from build123d import *

# Parameters (mm, degrees)
CROQUIS1_W              = 154.2
CROQUIS1_H              = 154.2
SALIENTE_EXTRUIR1_DEPTH = 0.8
CROQUIS2_R              = 60
CORTAR_EXTRUIR1_DEPTH   = 110.038800434
SALIENTE_EXTRUIR2_START = 1
CROQUIS3_R              = 60.995810587
CROQUIS3_R_2            = 60
SALIENTE_EXTRUIR2_DEPTH = 1
SALIENTE_EXTRUIR3_START = 0.5
CROQUIS4_R              = 62.434019261
CROQUIS4_R_2            = 60
SALIENTE_EXTRUIR3_DEPTH = 0.5
CROQUIS5_R              = 2.5
CROQUIS5_R_2            = 60
CORTAR_EXTRUIR2_DEPTH   = 110.046182877


with BuildPart() as part:
    # Croquis1 → Saliente-Extruir1 (new body)
    with BuildSketch(Plane(origin=(0, 0, 0), x_dir=(1, 0, 0), z_dir=(0, 1, 0))):
        Rectangle(CROQUIS1_W, CROQUIS1_H)
    extrude(amount=SALIENTE_EXTRUIR1_DEPTH)

    # Croquis2 → Cortar-Extruir1 (cut, through all)
    with BuildSketch(Plane(origin=(0, 0.8, 0), x_dir=(1, 0, 0), z_dir=(0, 1, 0))):
        with Locations(Location((0, 0, 0), (0, 0, 270))):
            Circle(CROQUIS2_R)
    extrude(amount=-CORTAR_EXTRUIR1_DEPTH, mode=Mode.SUBTRACT)

    # Croquis3 → Saliente-Extruir2 (add)
    with BuildSketch(Plane(origin=(0, 0.8, 0), x_dir=(1, 0, 0), z_dir=(0, 1, 0)).offset(SALIENTE_EXTRUIR2_START)):
        with Locations(Location((0, 0, 0), (0, 0, 90))):
            Circle(CROQUIS3_R)
        with Locations(Location((0, 0, 0), (0, 0, 270))):
            Circle(CROQUIS3_R_2, mode=Mode.SUBTRACT)
    extrude(amount=-SALIENTE_EXTRUIR2_DEPTH)

    # Croquis4 → Saliente-Extruir3 (add)
    with BuildSketch(Plane(origin=(0, 1.8, 0), x_dir=(1, 0, 0), z_dir=(0, 1, 0)).offset(SALIENTE_EXTRUIR3_START)):
        with Locations(Location((0, 0, 0), (0, 0, 270))):
            Circle(CROQUIS4_R)
        with Locations(Location((0, 0, 0), (0, 0, 270))):
            Circle(CROQUIS4_R_2, mode=Mode.SUBTRACT)
    extrude(amount=-SALIENTE_EXTRUIR3_DEPTH)

    # Croquis5 → Cortar-Extruir2 (cut, through all)
    with BuildSketch(Plane(origin=(0, 0.8, 0), x_dir=(1, 0, 0), z_dir=(0, 1, 0))):
        with Locations(Location((-59.39696962, 59.39696962, 0), (0, 0, 270))):
            Circle(CROQUIS5_R)
        with Locations(Location((-59.39696962, -59.39696962, 0), (0, 0, 90))):
            Circle(CROQUIS5_R)
        with Locations(Location((59.39696962, -59.39696962, 0), (0, 0, 270))):
            Circle(CROQUIS5_R)
        with Locations(Location((0, 0, 0), (0, 0, 270))):
            Circle(CROQUIS5_R_2)
        with Locations(Location((59.39696962, 59.39696962, 0), (0, 0, 90))):
            Circle(CROQUIS5_R)
    extrude(amount=-CORTAR_EXTRUIR2_DEPTH, mode=Mode.SUBTRACT)


solid = part.part
Source: CAD feature listing. Evaluate the final solid. Frame: model axes, mm. A direction names the side the tool comes from. Give positions to 0.01 mm unless a question says otherwise; leave off trailing zeros. Write each loop counter-clockwise with the first axis right and the second up, starting at its lowest first coordinate (ties: lowest second). Pieces come first, ordered by that corner, then holes. Notation, with made-up numbers: M 8.5,57 L 31.5,57 A32 ccw 31.5,90 Z; hole C 76,2.25 d3. An arc over 180 degrees is marked long. Return JSON: item names as keys, results as strings. Group by question number.
1) Draft query along Z for faces 3 (the face through (61.876, 0.406, 59.072)), 4 (the face through (37.12, 1.31, 48.4)), 5 (the face through (-60, 1.8, 14)). Return one class per face: released by +Z, released by -Z, zero draft, split by the parting line, or undercut.
2) Set-up query: faces 1 (the face through (-37.99, 2.053, -49.546)), 2 (the face through (33, 0, -52)). Return all of +Z, -Z, +X, -X, +Y, -Y with unobstructed straight access to the full face (end or side cutting, diameter ignored); none if empty.
3) Cut plane B-B, the plane x = 0. Output: boundary loops of the cut face in (y, z).
4) Ray query, L1, parallel to Z at x = 3.5, y = 1.6; L2, parallel to Z at x = 32.5, y = 1.9; L3, parallel to Y at x = -66.5, z = 22. Return the intervals inside material, ascending.
5) Cut plane A-A, the plane z = 0. Output: boundary loops of the cut face in (x, y), then the cut area to 3 significant figures.
6) First-contact query: pin 1 Ø8 at (x, z) = (-59.4, -59.4) entering from +Y. Flat tip, straight axial feed; report the tip coordinate or a pass-through.
Data:
{
 "1": {"face 3": "undercut", "face 4": "split by the parting line", "face 5": "zero draft"},
 "2": {"face 1": "+Y", "face 2": "+Z, -Z, +X, -X, -Y"},
 "3": {"outline": "M 0,-77.1 L 0.8,-77.1 L 0.8,-61 L 1.8,-61 L 1.8,-62.43 L 2.3,-62.43 L 2.3,-60 L 0,-60 Z; M 0,60 L 2.3,60 L 2.3,62.43 L 1.8,62.43 L 1.8,61 L 0.8,61 L 0.8,77.1 L 0,77.1 Z"},
 "4": {"L1": "z = -60.9 to -59.9, 59.9 to 60.9", "L2": "z = -53.31 to -50.44, 50.44 to 53.31", "L3": "y = 0 to 0.8"},
 "5": {"outline": "M -77.1,0 L -60,0 L -60,2.3 L -62.43,2.3 L -62.43,1.8 L -61,1.8 L -61,0.8 L -77.1,0.8 Z; M 60,0 L 77.1,0 L 77.1,0.8 L 61,0.8 L 61,1.8 L 62.43,1.8 L 62.43,2.3 L 60,2.3 Z", "area": "31.8 mm²"},
 "6": {"pin 1": "stops at y = 0.8"}
}
